from build123d import *

# Parameters (mm, degrees)
SKETCH2_W           = 14.8
SKETCH2_H           = 99.8
BOSS_EXTRUDE1_DEPTH = 10
BOSS_EXTRUDE2_START = -486.761258468
BOSS_EXTRUDE2_DEPTH = 270
SKETCH5_R           = 2.4
CUT_EXTRUDE1_DEPTH  = 4


# Read off the part's stored shape, not the designer's step: Boss-Extrude2
with BuildPart() as part:
    # Sketch2 → Boss-Extrude1 (new body)
    with BuildSketch(Plane.XY):
        with Locations((-106.280981946, -351.761258468)):
            Rectangle(SKETCH2_W, SKETCH2_H)
        with BuildLine():
            ThreePointArc((-103.980981946, -391.761258468), (-106.280981946, -389.461258468), (-108.580981946, -391.761258468))
            ThreePointArc((-108.580981946, -391.761258468), (-106.280981946, -394.061258468), (-103.980981946, -391.761258468))
        make_face(mode=Mode.SUBTRACT)
        with BuildLine():
            ThreePointArc((-108.580981946, -359.761258468), (-106.280981946, -362.061258468), (-103.980981946, -359.761258468))
            ThreePointArc((-103.980981946, -359.761258468), (-106.280981946, -357.461258468), (-108.580981946, -359.761258468))
        make_face(mode=Mode.SUBTRACT)
        with BuildLine():
            ThreePointArc((-108.580981946, -343.761258468), (-106.280981946, -346.061258468), (-103.980981946, -343.761258468))
            ThreePointArc((-103.980981946, -343.761258468), (-106.280981946, -341.461258468), (-108.580981946, -343.761258468))
        make_face(mode=Mode.SUBTRACT)
        with BuildLine():
            ThreePointArc((-108.580981946, -311.761258468), (-106.280981946, -314.061258468), (-103.980981946, -311.761258468))
            ThreePointArc((-103.980981946, -311.761258468), (-106.280981946, -309.461258468), (-108.580981946, -311.761258468))
        make_face(mode=Mode.SUBTRACT)
    extrude(amount=BOSS_EXTRUDE1_DEPTH)

    # Boss-Extrude2 outline → Boss-Extrude2 (add)
    with BuildSketch(Plane(origin=(0, 0, 0), x_dir=(1, 0, 0), z_dir=(0, 1, 0)).offset(BOSS_EXTRUDE2_START)):
        Polygon((-88.255797857, -7.152990504), (-88.255797857, 0), (-98.880981946, 0), (-98.880981946, -10), align=None)
    extrude(amount=BOSS_EXTRUDE2_DEPTH)

    # Sketch5 → Cut-Extrude1 (cut)
    with BuildSketch(Plane(origin=(-4.123769815, 0, -15.390118468), x_dir=(0.9659258262890692, 0, -0.25881904510251785), z_dir=(0.25881904510251785, 0, 0.9659258262890692))):
        with Locations((-92.599884641, -252.871258468)):
            Circle(SKETCH5_R)
        with Locations((-92.599884641, -450.651258468)):
            Circle(SKETCH5_R)
    extrude(amount=-CUT_EXTRUDE1_DEPTH, mode=Mode.SUBTRACT)


solid = part.part
The model under review builds one solid part; all positions refer to its coordinate system, in mm. A direction names the side the tool comes from. Give positions to 0.01 mm unless a question says otherwise; leave off trailing zeros. Write each loop counter-clockwise with the first axis right and the second up, starting at its lowest first coordinate (ties: lowest second). Pieces come first, ordered by that corner, then holes.
1. Add section C-C, the plane y = -438.5. Write out the cut boundary in (x, z), plus the area to 3 significant figures.
2. Wall thickness on L1, parallel to Y at x = -105, z = 9.75; L2, parallel to Y at x = -107.75, z = 0.75; L3, parallel to Y at x = -102.5, z = 1.75: over which ranges is each line inside the solid? List them lowest first.
3. For P1, Ø3, axis at x = -107.5, z = 6.5, coming from the -Y side; P2, Ø3, axis at x = -106.5, z = 6, coming from the +Y side; P3, Ø3, axis at y = -251, z = 5, coming from the -X side; P4, Ø6, axis at x = -106.28, y = -311.76, coming from the -Z side, all flat-tipped, find the tip position at first contact; note any pin that passes through.
4. Add section B-B, the plane y = -323. Write out the cut boundary in (x, z), plus the area to 3 significant figures.
5. Draft analysis for pull direction Z (two halves, no side actions). For faces 6 (the cylindrical face through (-94.38, -448.27, 6.75)), 7 (the flat face through (-94.636, -252.838, 4.721)), 8 (the flat face through (-113.681, -352, 5)), 9 (the flat face through (-93.643, -353.651, 8.596)), state which applies: +Z half, -Z half, draft (parallel to the pull), parting line (faces both ways), or undercut.
6. Tool access review of faces 1 (the flat face through (-106, -351, 10)), 2 (the flat face through (-98.881, -445, 5)), 3 (the flat face through (-98.881, -260, 5)), 4 (the flat face through (-94.636, -450.618, 4.721)), 5 (the flat face through (-98, -354, 0)): name each direction out of +Z, -Z, +X, -X, +Y, -Y from which nothing blocks a thin tool from reaching the whole face with its end or side.
7. Add section A-A, the plane z = 1.75. Write out the cut boundary in (x, y), plus the area to 3 significant figures.
Worked answers:
1. outline: (-98.88, 0) - (-88.26, 0) - (-88.26, 7.15) - (-98.88, 10) - close
1. area: 91.1 mm2
2. L1: y = -401.66 to -393.67, -389.85 to -361.67, -357.85 to -345.67, -341.85 to -313.67, -309.85 to -301.86
2. L2: y = -401.66 to -393.53, -389.99 to -361.53, -357.99 to -345.53, -341.99 to -313.53, -309.99 to -301.86
2. L3: y = -401.66 to -301.86
3. P1: stops at y = -401.66
3. P2: stops at y = -301.86
3. P3: stops at x = -98.88
3. P4: stops at z = 0
4. outline: (-113.68, 0) - (-88.26, 0) - (-88.26, 7.15) - (-98.88, 10) - (-113.68, 10) - close
4. area: 239 mm2
5. face 6: undercut
5. face 7: undercut
5. face 8: draft
5. face 9: +Z half
6. face 1: +Z, +X, -X, +Y, -Y
6. face 2: +Z, -Z, -X, -Y
6. face 3: +Z, -Z, -X, +Y
6. face 4: none
6. face 5: -Z, +X, -X, +Y, -Y
7. outline: (-113.68, -401.66) - (-98.88, -401.66) - (-98.88, -486.76) - (-88.26, -486.76) - (-88.26, -216.76) - (-98.88, -216.76) - (-98.88, -301.86) - (-113.68, -301.86) - close; hole circle Ø4.6 at (-106.28, -391.76); hole circle Ø4.6 at (-106.28, -359.76); hole circle Ø4.6 at (-106.28, -343.76); hole circle Ø4.6 at (-106.28, -311.76)
7. area: 4,280 mm2
